Can you work these out from the model? Positions are in its coordinate system, mm. A direction names the side the tool comes from. Round coordinates to 2 decimals unless told otherwise and drop trailing zeros. Loops run counter-clockwise (first coordinate to the right, second up) from the corner with the lowest first, then second, coordinate; pieces in that order, holes last.
```python
from build123d import *

# Parameters (mm, degrees)
F0_W     = 3
F0_H     = 13
F0_H_2   = 2
F0_W_2   = 27
F0_H_3   = 4
F1_DEPTH = 22
F0_W_3   = 7
F0_H_4   = 11.0040441751
F2_DEPTH = 2
F3_R     = 4.25
F4_DEPTH = 40
F5_R     = 5


with BuildPart() as f1:
    # F0 (on Top) → F1 (new body)
    with BuildSketch(Plane.XY):
        Polygon((3, 30), (0, 30), (0, 19), (3, 19), (3, 28), align=None)
        Polygon((33, 30), (3, 30), (3, 28), (30, 28), (33, 28), align=None)
        with Locations((31.5, 21.5)):
            Rectangle(F0_W, F0_H)
        with Locations((31.5, 8.5)):
            Rectangle(F0_W, F0_H)
        with Locations((31.5, 1)):
            Rectangle(F0_W, F0_H_2)
        with Locations((16.5, 1)):
            Rectangle(F0_W_2, F0_H_2)
        Polygon((3, 11), (0, 11), (0, 0), (3, 0), (3, 2), align=None)
        with Locations((1.5, 13)):
            Rectangle(F0_W, F0_H_3)
        with Locations((1.5, 17)):
            Rectangle(F0_W, F0_H_3)
    extrude(amount=F1_DEPTH)

    # F0 (on Top) → F2 (join)
    with BuildSketch(Plane.XY):
        Polygon((30, 28), (3, 28), (3, 19), (3, 15), (6.5, 15), (6.5, 26.0040441751), (13.5, 26.0040441751), (13.5, 15), (16.5, 15), (19.5, 15), (19.5, 26.0040441751), (26.5, 26.0040441751), (26.5, 15), (30, 15), align=None)
        Polygon((6.5, 15), (3, 15), (3, 11), (3, 2), (30, 2), (30, 15), (26.5, 15), (26.5, 3.9959558249), (19.5, 3.9959558249), (19.5, 15), (16.5, 15), (13.5, 15), (13.5, 3.9959558249), (6.5, 3.9959558249), align=None)
        with Locations((10, 9.4979779124)):
            Rectangle(F0_W_3, F0_H_4)
        with Locations((10, 20.5020220876)):
            Rectangle(F0_W_3, F0_H_4)
        with Locations((23, 20.5020220876)):
            Rectangle(F0_W_3, F0_H_4)
        with Locations((23, 9.4979779124)):
            Rectangle(F0_W_3, F0_H_4)
    extrude(amount=F2_DEPTH)

    # F3 (on Right) → F4 (cut)
    with BuildSketch(Plane.YZ):
        with Locations((15, 16)):
            Circle(F3_R)
    extrude(amount=F4_DEPTH, mode=Mode.SUBTRACT)

    # F5
    f5_edges = [f1.edges().sort_by_distance(p)[0] for p in [
        (16.5, 30, 0),
        (0, 15, 0),
        (16.5, 0, 0),
        (33, 15, 0),
        (33, 30, 11),
        (0, 30, 11),
        (0, 0, 11),
        (33, 0, 11),
    ]]
    fillet(f5_edges, radius=F5_R)


solid = f1.part
```
(1) For pin 1 (8 mm diameter, centred on x = 17.5, y = 13, fed in from +Z), with a flat end and sliding along its axis, tell me the tip position at first contact or that it passes through.
(2) Suppose I cut it at D-D (y = 21.5). Write out the boundary of the cut face in (x, z), then the cut area to 3 significant figures.
(3) Suppose I cut it at A-A (z = 10.5). Write out the boundary of the cut face in (x, y).
(4) Suppose I cut it at B-B (y = 15). Write out the boundary of the cut face in (x, z).
(5) We'd pull the mould along Y, two halves only. Please class faces 1 (the flat face through (17, 30, 13)), 2 (the cylindrical face through (31.48, 14.08, 11.85)), 3 (the cylindrical face through (1, 2, 14)): released by +Y, released by -Y, zero draft, split by the parting line, or undercut.
(6) Suppose I cut it at C-C (z = 16). Write out the boundary of the cut face in (x, y).
(7) If I drill on line 1 (X direction, y = 19, z = 7.5); line 2 (Y direction, x = 16.5, z = 17); line 3 (X direction, y = 27.25, z = 18.5), over which ranges is the centre line in solid material (lowest first)?
(8) Which directions (+Z, -Z, +X, -X, +Y, -Y) give clear straight access to the entire face, cutting with the end or side of a thin tool? Please do faces 4 (the flat face through (16, 15, 2)), 5 (the flat face through (16, 0, 13)).
Check result:
1. pin 1: stops at z = 2
2. outline: (0, 5) arc R5 ccw to (5, 0) - (28, 0) arc R5 ccw to (33, 5) - (33, 22) - (30, 22) - (30, 2) - (3, 2) - (3, 22) - (0, 22) - close
2. area: 175 mm2
3. outline: (0, 5) arc R5 ccw to (5, 0) - (28, 0) arc R5 ccw to (33, 5) - (33, 25) arc R5 ccw to (28, 30) - (5, 30) arc R5 ccw to (0, 25) - close; hole (3, 2) - (30, 2) - (30, 28) - (3, 28) - close
4. outline: (0, 5) arc R5 ccw to (5, 0) - (28, 0) arc R5 ccw to (33, 5) - (33, 11.75) - (30, 11.75) - (30, 2) - (3, 2) - (3, 11.75) - (0, 11.75) - close; (0, 20.25) - (3, 20.25) - (3, 22) - (0, 22) - close; (30, 20.25) - (33, 20.25) - (33, 22) - (30, 22) - close
5. face 1: released by +Y
5. face 2: undercut
5. face 3: released by -Y
6. outline: (0, 5) arc R5 ccw to (5, 0) - (28, 0) arc R5 ccw to (33, 5) - (33, 10.75) - (30, 10.75) - (30, 2) - (3, 2) - (3, 10.75) - (0, 10.75) - close; (0, 19.25) - (3, 19.25) - (3, 28) - (30, 28) - (30, 19.25) - (33, 19.25) - (33, 25) arc R5 ccw to (28, 30) - (5, 30) arc R5 ccw to (0, 25) - close
7. line 1: x = 0 to 3, 30 to 33
7. line 2: y = 0 to 2, 28 to 30
7. line 3: x = 0.53 to 3, 30 to 32.47
8. face 4: +Z
8. face 5: +Z, -Z, +X, -X, -Y
